Work out the finished part from the listing and answer in its coordinate system (mm). Face numbers are marked on the shaded views. A direction names the side the tool comes from. Round coordinates to 2 decimals unless told otherwise and drop trailing zeros. Loops run counter-clockwise (first coordinate to the right, second up) from the corner with the lowest first, then second, coordinate; pieces in that order, holes last. Notation, with made-up numbers: (9.25, 31) - (37.25, 31) arc R17 cw to (37.25, 38) - close; hole circle Ø9 at (-23, 68.5). An arc over 180 degrees is marked (long way). Return JSON: item names as keys, results as strings.
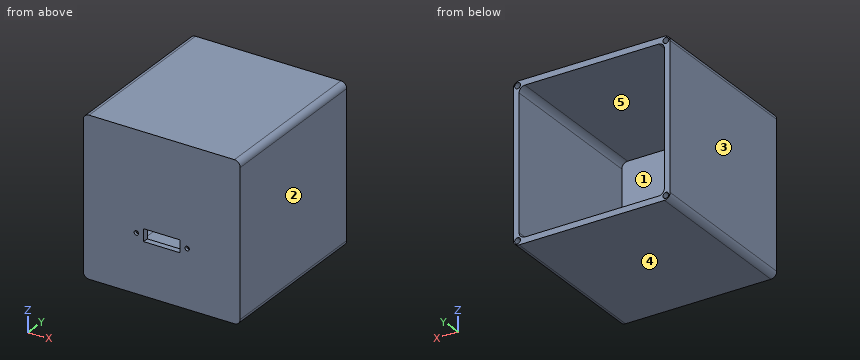
from build123d import *

# Parameters (mm, degrees)
F0_W      = 137.16
F0_H      = 137.16
F1_DEPTH  = 5.08
F2_W      = 5.08
F2_H      = 127
F3_DEPTH  = 139.7
F4_W      = 15.875
F4_H      = 10.795
F5_DEPTH  = 5.08
F6_R      = 1.905
F7_DEPTH  = 5.08
F8_R      = 5.08
F10_DEPTH = 2.54
F12_DEPTH = 22.86


with BuildPart() as f1:
    # F0 (on Front) → F1 (new body)
    with BuildSketch(Plane.XZ):
        with Locations((68.58, 68.58)):
            Rectangle(F0_W, F0_H)
    extrude(amount=F1_DEPTH)

    # F2 (on face) → F3 (join)
    with BuildSketch(Plane(origin=(0, 0, 0), x_dir=(-1, 0, 0), z_dir=(0, 1, 0))):
        Polygon((-132.08, 137.16), (-137.16, 137.16), (-137.16, 0), (-132.08, 0), (-132.08, 5.08), (-132.08, 132.08), align=None)
        Polygon((0, 137.16), (-132.08, 137.16), (-132.08, 132.08), (-5.08, 132.08), (0, 132.08), align=None)
        Polygon((-132.08, 5.08), (-132.08, 0), (0, 0), (0, 5.08), (-5.08, 5.08), align=None)
        with Locations((-2.54, 68.58)):
            Rectangle(F2_W, F2_H)
    extrude(amount=F3_DEPTH)

    # F4 (on face) → F5 (cut, through all)
    with BuildSketch(Plane.XZ.offset(5.08)):
        with Locations((76.5175, 50.8)):
            Rectangle(F4_W, F4_H)
        with Locations((60.6425, 50.8)):
            Rectangle(F4_W, F4_H)
    extrude(amount=-F5_DEPTH, mode=Mode.SUBTRACT)

    # F6 (on face) → F7 (cut, through all)
    with BuildSketch(Plane.XZ.offset(5.08)):
        with BuildLine():
            ThreePointArc((88.9, 50.8), (90.805, 48.895), (92.71, 50.8))
            ThreePointArc((92.71, 50.8), (90.805, 52.705), (88.9, 50.8))
        make_face()
        with Locations((46.355, 50.8)):
            Circle(F6_R)
    extrude(amount=-F7_DEPTH, mode=Mode.SUBTRACT)

    # F8
    f8_edges = [f1.edges().sort_by_distance(p)[0] for p in [
        (0, 67.31, 137.16),
        (137.16, 67.31, 137.16),
        (0, 67.31, 0),
        (137.16, 67.31, 0),
        (5.08, 69.85, 132.08),
        (132.08, 69.85, 132.08),
        (5.08, 69.85, 5.08),
        (132.08, 69.85, 5.08),
    ]]
    fillet(f8_edges, radius=F8_R)

    # F9 (on face) → F10 (cut)
    with BuildSketch(Plane(origin=(0, 0, 0), x_dir=(-1, 0, 0), z_dir=(0, 1, 0))):
        Polygon((-89.0524, 53.835592), (-92.5576, 53.835592), (-94.3102, 50.8), (-92.5576, 47.764408), (-89.0524, 47.764408), (-87.2998, 50.8), align=None)
        Polygon((-42.8498, 50.8), (-44.6024, 53.835592), (-48.1076, 53.835592), (-49.8602, 50.8), (-48.1076, 47.764408), (-44.6024, 47.764408), align=None)
    extrude(amount=-F10_DEPTH, mode=Mode.SUBTRACT)

    # F11 (on face) → F12 (cut)
    with BuildSketch(Plane(origin=(0, 139.7, 0), x_dir=(-1, 0, 0), z_dir=(0, 1, 0))):
        with BuildLine():
            Line((-133.35, 130.81), (-133.35, 133.35))
            Line((-133.35, 133.35), (-130.81, 133.35))
            ThreePointArc((-130.81, 133.35), (-135.146051, 135.146051), (-133.35, 130.81))
        make_face()
        with BuildLine():
            Line((-130.81, 133.35), (-133.35, 133.35))
            Line((-133.35, 133.35), (-133.35, 130.81))
            ThreePointArc((-133.35, 130.81), (-131.553949, 131.553949), (-130.81, 133.35))
        make_face()
        with BuildLine():
            ThreePointArc((-130.81, 3.81), (-131.553949, 5.606051), (-133.35, 6.35))
            Line((-133.35, 6.35), (-133.35, 3.81))
            Line((-133.35, 3.81), (-130.81, 3.81))
        make_face()
        with BuildLine():
            Line((-133.35, 3.81), (-133.35, 6.35))
            ThreePointArc((-133.35, 6.35), (-135.146051, 2.013949), (-130.81, 3.81))
            Line((-130.81, 3.81), (-133.35, 3.81))
        make_face()
        with BuildLine():
            Line((-3.81, 3.81), (-3.81, 6.35))
            ThreePointArc((-3.81, 6.35), (-5.606051, 5.606051), (-6.35, 3.81))
            Line((-6.35, 3.81), (-3.81, 3.81))
        make_face()
        with BuildLine():
            ThreePointArc((-1.27, 3.81), (-2.013949, 5.606051), (-3.81, 6.35))
            Line((-3.81, 6.35), (-3.81, 3.81))
            Line((-3.81, 3.81), (-6.35, 3.81))
            ThreePointArc((-6.35, 3.81), (-3.81, 1.27), (-1.27, 3.81))
        make_face()
        with BuildLine():
            Line((-3.81, 133.35), (-6.35, 133.35))
            ThreePointArc((-6.35, 133.35), (-5.606051, 131.553949), (-3.81, 130.81))
            Line((-3.81, 130.81), (-3.81, 133.35))
        make_face()
        with BuildLine():
            ThreePointArc((-1.27, 133.35), (-3.81, 135.89), (-6.35, 133.35))
            Line((-6.35, 133.35), (-3.81, 133.35))
            Line((-3.81, 133.35), (-3.81, 130.81))
            ThreePointArc((-3.81, 130.81), (-2.013949, 131.553949), (-1.27, 133.35))
        make_face()
    extrude(amount=-F12_DEPTH, mode=Mode.SUBTRACT)


solid = f1.part
1) Section D-D (z = 116) is taken. Give the vertices of the cut face in (x, y).
Verdict:
{"outline": "(0, -5.08) - (137.16, -5.08) - (137.16, 139.7) - (132.08, 139.7) - (132.08, 0) - (5.08, 0) - (5.08, 139.7) - (0, 139.7) - close"}
2) Flat-ended cylindrical pins translate along their axes: pin 1 (3.5 mm diameter, centred on x = 90.805, z = 50.8, fed in from -Y); pin 2 (2.5 mm diameter, centred on x = 3, z = 4, fed in from +Y); pin 3 (12 mm diameter, centred on x = 60, z = 68.5, fed in from +Y). Find the tip coordinate at first contact, or state that the pin passes through.
Verdict:
{"pin 1": "passes through", "pin 2": "stops at y = 116.84", "pin 3": "stops at y = 0"}
3) Section A-A (x = 70.5) is taken. Give the vertices of the cut face in (y, z), and give its area (3 significant figures).
Verdict:
{"outline": "(-5.08, 0) - (139.7, 0) - (139.7, 5.08) - (0, 5.08) - (0, 45.4) - (-5.08, 45.4) - close; (-5.08, 56.2) - (0, 56.2) - (0, 132.08) - (139.7, 132.08) - (139.7, 137.16) - (-5.08, 137.16) - close", "area": "2,060 mm2"}
4) Section C-C (x = 19) is taken. Give the vertices of the cut face in (y, z).
Verdict:
{"outline": "(-5.08, 0) - (139.7, 0) - (139.7, 5.08) - (0, 5.08) - (0, 132.08) - (139.7, 132.08) - (139.7, 137.16) - (-5.08, 137.16) - close"}
5) Find the intervals of material crossed by L1, parallel to X at y = 107, z = 84; L2, parallel to X at y = 132.5, z = 133.35, in increasing order.
Verdict:
{"L1": "x = 0 to 5.08, 132.08 to 137.16", "L2": "x = 0.16 to 1.27, 6.35 to 130.81, 135.89 to 137"}
6) A tool of negligible diameter and unlimited length cuts with its end or side. For the marked faces 4 and 5, from which of +Z, -Z, +X, -X, +Y, -Y can it reach the whole face along a straight path? Write none if from no direction.
Verdict:
{"face 4": "-Z, +X, -X, +Y, -Y", "face 5": "+Y"}
7) Determine the mould class of the marked faces 1, 2 and 3 for opening direction X: pulls with the +X half, pulls with the -X half, needs draft (parallel to the pull), parting line crosses it, or undercut.
Verdict:
{"face 1": "undercut", "face 2": "pulls with the +X half", "face 3": "pulls with the -X half"}
8) Section B-B (y = 18.5) is taken. Give the vertices of the cut face in (x, z), and give its area (3 significant figures).
Verdict:
{"outline": "(0, 5.08) arc R5.08 ccw to (5.08, 0) - (132.08, 0) arc R5.08 ccw to (137.16, 5.08) - (137.16, 132.08) arc R5.08 ccw to (132.08, 137.16) - (5.08, 137.16) arc R5.08 ccw to (0, 132.08) - close; hole (5.08, 10.16) arc R5.08 ccw to (10.16, 5.08) - (127, 5.08) arc R5.08 ccw to (132.08, 10.16) - (132.08, 127) arc R5.08 ccw to (127, 132.08) - (10.16, 132.08) arc R5.08 ccw to (5.08, 127) - close", "area": "2,680 mm2"}
